Geometry: final body of the model. Coordinates: model frame, mm. A direction names the side the tool comes from. Give positions to 0.01 mm unless a question says otherwise; leave off trailing zeros. Write each loop counter-clockwise with the first axis right and the second up, starting at its lowest first coordinate (ties: lowest second). Pieces come first, ordered by that corner, then holes. Notation, with made-up numbers: M 33,71.25 L 85,71.25 A27 cw 85,89.25 Z; hole C 22,81.25 d2. An arc over 180 degrees is marked long. One line per question, with ' | ' between items.
from build123d import *

# Parameters (mm, degrees)
BOSS_EXTRUDE1_DEPTH        = 30
SKETCH2_W                  = 10
SKETCH2_H                  = 20
CUT_EXTRUDE1_DEPTH         = 30
SKETCH3_R                  = 40
BOSS_EXTRUDE2_DEPTH        = 40
SKETCH4_R                  = 25
BOSS_EXTRUDE3_DEPTH        = 20
CUT_EXTRUDE2_DEPTH         = 42
CUT_EXTRUDE3_DEPTH         = 42
BOSS_EXTRUDE4_DEPTH        = 10
BOSS_EXTRUDE5_DEPTH        = 10
SKETCH9_R                  = 5
CUT_EXTRUDE4_DEPTH         = 10
CUT_EXTRUDE5_DEPTH         = 20
CUT_EXTRUDE5_DEPTH_BACK    = 20
SKETCH11_R                 = 5
CUT_EXTRUDE6_DEPTH         = 50
F_20_0MM_DOWEL_HOLE1_D     = 20
F_20_0MM_DOWEL_HOLE1_DEPTH = 30
F_20_0MM_DOWEL_HOLE1_TIP   = 6.00860619


with BuildPart() as part:
    # Sketch1 → Boss-Extrude1 (new body)
    with BuildSketch(Plane.XY):
        with BuildLine():
            ThreePointArc((90, 100), (140, 50), (90, 0))
            Line((90, 0), (0, 0))
            Line((0, 0), (0, 100))
            Line((0, 100), (90, 100))
        make_face()
    extrude(amount=BOSS_EXTRUDE1_DEPTH)

    # Sketch2 → Cut-Extrude1 (cut)
    with BuildSketch(Plane.XY.offset(30)):
        with BuildLine():
            Line((0, 90), (0, 100))
            Line((0, 100), (10, 100))
            ThreePointArc((10, 100), (2.928932188, 97.071067812), (0, 90))
        make_face()
        with BuildLine():
            Line((0, 10), (0, 0))
            Line((0, 0), (10, 0))
            ThreePointArc((10, 0), (2.928932188, 2.928932188), (0, 10))
        make_face()
        with Locations((5, 70)):
            Rectangle(SKETCH2_W, SKETCH2_H)
        with Locations((5, 30)):
            Rectangle(SKETCH2_W, SKETCH2_H)
    extrude(amount=-CUT_EXTRUDE1_DEPTH, mode=Mode.SUBTRACT)

    # Sketch3 → Boss-Extrude2 (add)
    with BuildSketch(Plane.XY.offset(30)):
        with Locations((90, 50)):
            Circle(SKETCH3_R)
    extrude(amount=BOSS_EXTRUDE2_DEPTH)

    # Sketch4 → Boss-Extrude3 (add)
    with BuildSketch(Plane.XY.offset(70)):
        with Locations((90, 50)):
            Circle(SKETCH4_R)
    extrude(amount=BOSS_EXTRUDE3_DEPTH)

    # Sketch5 → Cut-Extrude2 (cut)
    with BuildSketch(Plane.XY.offset(30)):
        with BuildLine():
            ThreePointArc((20, 80), (30, 70), (20, 60))
            Line((20, 60), (10, 60))
            Line((10, 60), (10, 80))
            Line((10, 80), (20, 80))
        make_face()
    extrude(amount=-CUT_EXTRUDE2_DEPTH, mode=Mode.SUBTRACT)

    # Sketch6 → Cut-Extrude3 (cut)
    with BuildSketch(Plane.XY.offset(30)):
        with BuildLine():
            ThreePointArc((20, 40), (30, 30), (20, 20))
            Line((20, 20), (10, 20))
            Line((10, 20), (10, 40))
            Line((10, 40), (20, 40))
        make_face()
    extrude(amount=-CUT_EXTRUDE3_DEPTH, mode=Mode.SUBTRACT)

    # Sketch7 → Boss-Extrude4 (add)
    with BuildSketch(Plane.XY.offset(10)):
        with BuildLine():
            Line((10, 80), (10, 60))
            Line((10, 60), (20, 60))
            ThreePointArc((20, 60), (30, 70), (20, 80))
            Line((20, 80), (10, 80))
        make_face()
    extrude(amount=BOSS_EXTRUDE4_DEPTH)

    # Sketch8 → Boss-Extrude5 (add)
    with BuildSketch(Plane.XY.offset(10)):
        with BuildLine():
            Line((10, 40), (10, 20))
            Line((10, 20), (20, 20))
            ThreePointArc((20, 20), (30, 30), (20, 40))
            Line((20, 40), (10, 40))
        make_face()
    extrude(amount=BOSS_EXTRUDE5_DEPTH)

    # Sketch9 → Cut-Extrude4 (cut)
    with BuildSketch(Plane.XY.offset(20)):
        with Locations((20, 70)):
            Circle(SKETCH9_R)
        with Locations((20, 30)):
            Circle(SKETCH9_R)
    extrude(amount=-CUT_EXTRUDE4_DEPTH, mode=Mode.SUBTRACT)

    # Sketch10 → Cut-Extrude5 (cut, two sides)
    with BuildSketch(Plane.XY.offset(70)) as cut_extrude5_sk:
        with BuildLine():
            ThreePointArc((63.542486889, 20), (73.542486889, 50), (63.542486889, 80))
            Line((63.542486889, 80), (63.542486889, 20))
        make_face()
        with BuildLine():
            Line((63.542486889, 20), (63.542486889, 80))
            ThreePointArc((63.542486889, 80), (50, 50), (63.542486889, 20))
        make_face()
    extrude(amount=CUT_EXTRUDE5_DEPTH, mode=Mode.SUBTRACT)
    extrude(cut_extrude5_sk.sketch, amount=-CUT_EXTRUDE5_DEPTH_BACK, mode=Mode.SUBTRACT)

    # Sketch11 → Cut-Extrude6 (cut)
    with BuildSketch(Plane.XY.offset(50)):
        with Locations((60, 50)):
            Circle(SKETCH11_R)
    extrude(amount=-CUT_EXTRUDE6_DEPTH, mode=Mode.SUBTRACT)

    # 20.0mm Dowel Hole1
    with Locations(Plane(origin=(90, 50, 90), x_dir=(1, 0, 0), z_dir=(0, 0, 1))):
        with Locations((0, 0)):
            Hole(F_20_0MM_DOWEL_HOLE1_D / 2, depth=F_20_0MM_DOWEL_HOLE1_DEPTH)
            with Locations((0, 0, -(F_20_0MM_DOWEL_HOLE1_DEPTH + F_20_0MM_DOWEL_HOLE1_TIP / 2))):  # 118° drill point
                Cone(0, F_20_0MM_DOWEL_HOLE1_D / 2, F_20_0MM_DOWEL_HOLE1_TIP, mode=Mode.SUBTRACT)


solid = part.part
(1) Cut plane D-D, the plane y = 30. Return loops of the section in (x, z), then the cut area to 3 significant figures.
Working result:
outline: M 10,10 L 15,10 L 15,20 L 10,20 Z; M 25,10 L 30,10 L 30,0 L 135.83,0 L 135.83,30 L 124.64,30 L 124.64,70 L 105,70 L 105,90 L 75,90 L 75,70 L 69.37,70 L 69.37,50 L 55.36,50 L 55.36,30 L 30,30 L 30,20 L 25,20 Z | area: 6,370 mm^2
(2) Cut plane A-A, the plane z = 6. Return loops of the section in (x, y).
Working result:
outline: M 0,10 A10 ccw 10,0 L 90,0 A50 ccw 90,100 L 10,100 A10 ccw 0,90 L 0,80 L 20,80 A10 cw 20,60 L 0,60 L 0,40 L 20,40 A10 cw 20,20 L 0,20 Z; hole C 60,50 d10
(3) Draft query along Y for faces 6 (the face through (0, 15, 15)), 7 (the face through (59.349, 54.957, 25.35)), 8 (the face through (126.95, 34.68, 49.72)), 9 (the face through (49, 100, 15)). Return one class per face: released by +Y, released by -Y, zero draft, split by the parting line, or undercut.
Working result:
face 6: zero draft | face 7: undercut | face 8: split by the parting line | face 9: released by +Y
(4) First-contact query: P1, Ø11.5, axis at x = 20, y = 70, coming from the +Z side; P2, Ø3, axis at x = 43, y = 47, coming from the +Z side; P3, Ø12, axis at y = 40, z = 30, coming from the +X side; P4, Ø23, axis at x = 90, y = 50, coming from the +Z side. Flat tips, straight axial feed; report the tip coordinate or a pass-through.
Working result:
P1: stops at z = 20 | P2: stops at z = 30 | P3: stops at x = 139.84 | P4: stops at z = 90
(5) Cut plane B-B, the plane x = 61.5. Return loops of the section in (y, z).
Working result:
outline: M 0,0 L 45.23,0 L 45.23,50 L 21.93,50 L 21.93,30 L 0,30 Z; M 54.77,0 L 100,0 L 100,30 L 78.07,30 L 78.07,50 L 54.77,50 Z
(6) Cut plane C-C, the plane z = 17. Return loops of the section in (x, y), then the cut area to 3 significant figures.
Working result:
outline: M 0,10 A10 ccw 10,0 L 90,0 A50 ccw 90,100 L 10,100 A10 ccw 0,90 L 0,80 L 10,80 L 10,60 L 0,60 L 0,40 L 10,40 L 10,20 L 0,20 Z; hole C 20,30 d10; hole C 20,70 d10; hole C 60,50 d10 | area: 12,200 mm^2
(7) Material intervals for L1, parallel to Y at x = 20, z = 18; L2, parallel to X at y = 50, z = 72; L3, parallel to Y at x = 60, z = 15.5, sorted ascending. Write a range as [from, to].
Working result:
L1: y = [0, 25], [35, 65], [75, 100] | L2: x = [73.54, 80], [100, 115] | L3: y = [0, 45], [55, 100]
(8) Set-up query: faces 1 (the face through (8, 20, 15)), 2 (the face through (10, 70, 15)), 3 (the face through (40, 51, 30)), 4 (the face through (15, 68, 10)), 5 (the face through (30, 70, 25)). Return all of +Z, -Z, +X, -X, +Y, -Y with unobstructed straight access to the full face (end or side cutting, diameter ignored); none if empty.
Working result:
face 1: -X | face 2: +Z, -Z, -X | face 3: +Z | face 4: -Z, -X | face 5: +Z, -X
